Work out the finished part from the listing and answer in its coordinate system (mm). A direction names the side the tool comes from. Coordinates: 2 decimals unless noted, no trailing zeros. Loops run counter-clockwise (first coordinate to the right, second up) from the corner with the lowest first, then second, coordinate; pieces in that order, holes last. Notation, with made-up numbers: (18.25, 83) - (62.25, 83) arc R29 ccw to (62.25, 107) - close; hole circle Ø3 at (2, 30). An arc over 180 degrees is marked (long way). Write each question's results on one line, items separated by ' | '. Start each with the question number.
Item 1: Each of these flat-tipped pins is pushed along its axis until it touches: pin 1 Ø1 at (y, z) = (20, 1) entering from +X; pin 2 Ø3 at (x, z) = (101, 3.5) entering from -Y. Where does it stop, or does it pass through?
Item 2: Consider probe 1 along X at (y, z) = (67.5, 4.9); probe 2 along X at (y, z) = (36.5, 1.3); probe 3 along X at (y, z) = (90.29, 2.85). Determine where each line is inside the solid, lowest interval first. Write a range as [from, to].
Item 3: Section A-A, the plane x = 69 is taken. Write down the section's boundary in (y, z) (3 decimals), plus the area to 4 significant figures.
Item 4: A tool of negligible diameter and unlimited length cuts with its end or side. For faces 1 (the face through (145, 16.73, 3)), 2 (the face through (35, 90.73, 3)), 3 (the face through (-89, -35, 3)), from which of +Z, -Z, +X, -X, +Y, -Y can it reach the whole face along a straight path? Write none if from no direction.
Item 5: Section C-C, the plane z = 1.05 is taken. Count the separate pieces of the cut face and the enclosed holes in it, plus the area to 3 significant figures.
Item 6: For a pull along Y with two mould halves and no side action, classify faces 4 (the face through (-109, -35, 3)), 5 (the face through (-162, 83.853, 3)), 6 (the face through (-105, 90.73, 3)) as +Y half, -Y half, draft (parallel to the pull), parting line (faces both ways), or undercut.
Item 7: Section B-B, the plane y = 31 is taken. Write down the section's boundary in (x, z), plus the area to 3 significant figures.
from build123d import *

# Parameters (mm, degrees)
BOSS_EXTRU_1_DEPTH      = 6
ESQUISSE3_W             = 6
ESQUISSE3_H             = 10
ESQUISSE3_W_2           = 20
ESQUISSE3_H_2           = 6
ESQUISSE3_W_3           = 60
ESQUISSE3_H_3           = 110
ESQUISSE3_W_4           = 40
ESQUISSE3_H_4           = 20
ENL_V_MAT_EXTRU_2_DEPTH = 6
ESQUISSE4_R             = 1.5
ENL_V_MAT_EXTRU_3_DEPTH = 6
ESQUISSE5_W             = 456.045253014
ESQUISSE5_H             = 136.228984631
ENL_V_MAT_EXTRU_4_DEPTH = 6


with BuildPart() as part:
    # Esquisse1 → Boss.-Extru.1 (new body)
    with BuildSketch(Plane.XY):
        Polygon((-165, 96.73), (165, 96.73), (165, -18.27), (123, -109.022410436), (-123, -109.022410436), (-165, -18.27), align=None)
    extrude(amount=BOSS_EXTRU_1_DEPTH)

    # Esquisse3 → Enlèv. mat.-Extru.2 (cut)
    with BuildSketch(Plane(origin=(0, 0, 0), x_dir=(-1, 0, 0), z_dir=(0, 0, -1))):
        with Locations((162, -4.85)):
            Rectangle(ESQUISSE3_W, ESQUISSE3_H)
        with Locations((162, 78.852589564)):
            Rectangle(ESQUISSE3_W, ESQUISSE3_H)
        with Locations((-24, -35.02)):
            Rectangle(ESQUISSE3_W_2, ESQUISSE3_H_2)
        with Locations((99, -35.02)):
            Rectangle(ESQUISSE3_W_2, ESQUISSE3_H_2)
        with Locations((-162, 51.23)):
            Rectangle(ESQUISSE3_W, ESQUISSE3_H)
        with Locations((-80, 29.355)):
            Rectangle(ESQUISSE3_W_3, ESQUISSE3_H_3)
        with Locations((24, -35.02)):
            Rectangle(ESQUISSE3_W_2, ESQUISSE3_H_2)
        with Locations((-162, 78.852589564)):
            Rectangle(ESQUISSE3_W, ESQUISSE3_H)
        with Locations((-162, -4.85)):
            Rectangle(ESQUISSE3_W, ESQUISSE3_H)
        with Locations((105, 93.73)):
            Rectangle(ESQUISSE3_W_2, ESQUISSE3_H_2)
        with Locations((-35, 93.73)):
            Rectangle(ESQUISSE3_W_2, ESQUISSE3_H_2)
        with Locations((35, 93.73)):
            Rectangle(ESQUISSE3_W_2, ESQUISSE3_H_2)
        with Locations((-105, 93.73)):
            Rectangle(ESQUISSE3_W_2, ESQUISSE3_H_2)
        with Locations((162, 51.23)):
            Rectangle(ESQUISSE3_W, ESQUISSE3_H)
        with Locations((-99, -35.02)):
            Rectangle(ESQUISSE3_W_2, ESQUISSE3_H_2)
        with Locations((-145, 26.73)):
            Rectangle(ESQUISSE3_W_4, ESQUISSE3_H_4)
        with Locations((145, 26.73)):
            Rectangle(ESQUISSE3_W_4, ESQUISSE3_H_4)
    extrude(amount=-ENL_V_MAT_EXTRU_2_DEPTH, mode=Mode.SUBTRACT)

    # Esquisse4 → Enlèv. mat.-Extru.3 (cut)
    with BuildSketch(Plane(origin=(0, 0, 0), x_dir=(-1, 0, 0), z_dir=(0, 0, -1))):
        with Locations((162, 7.65)):
            Circle(ESQUISSE4_R)
        with Locations((114, -35.02)):
            Circle(ESQUISSE4_R)
        with Locations((162, 65.042589564)):
            Circle(ESQUISSE4_R)
        with Locations((84, -35.02)):
            Circle(ESQUISSE4_R)
        with Locations((39, -35.02)):
            Circle(ESQUISSE4_R)
        with Locations((162, 90.29)):
            Circle(ESQUISSE4_R)
        with Locations((9, -35.02)):
            Circle(ESQUISSE4_R)
        with Locations((-9, -35.02)):
            Circle(ESQUISSE4_R)
        with Locations((-39, -35.02)):
            Circle(ESQUISSE4_R)
        with Locations((-84, -35.02)):
            Circle(ESQUISSE4_R)
        with Locations((120, 93.73)):
            Circle(ESQUISSE4_R)
        with Locations((-114, -35.02)):
            Circle(ESQUISSE4_R)
        with Locations((90, 93.73)):
            Circle(ESQUISSE4_R)
        with Locations((50, 93.73)):
            Circle(ESQUISSE4_R)
        with Locations((20, 93.73)):
            Circle(ESQUISSE4_R)
        with Locations((-20, 93.73)):
            Circle(ESQUISSE4_R)
        with Locations((-50, 93.73)):
            Circle(ESQUISSE4_R)
        with Locations((-90, 93.73)):
            Circle(ESQUISSE4_R)
        with Locations((-120, 93.73)):
            Circle(ESQUISSE4_R)
        with Locations((-162, 90.29)):
            Circle(ESQUISSE4_R)
        with Locations((-162, 65.042589564)):
            Circle(ESQUISSE4_R)
        with Locations((-162, 7.65)):
            Circle(ESQUISSE4_R)
    extrude(amount=-ENL_V_MAT_EXTRU_3_DEPTH, mode=Mode.SUBTRACT)

    # Esquisse5 → Enlèv. mat.-Extru.4 (cut)
    with BuildSketch(Plane(origin=(0, 0, 0), x_dir=(-1, 0, 0), z_dir=(0, 0, -1))):
        with Locations((-18.307092018, -106.134492316)):
            Rectangle(ESQUISSE5_W, ESQUISSE5_H)
    extrude(amount=-ENL_V_MAT_EXTRU_4_DEPTH, mode=Mode.SUBTRACT)


solid = part.part
Answer key:
1) pin 1: stops at x = 125 | pin 2: stops at y = -32.02
2) probe 1: x = [-165, 50], [110, 165] | probe 2: x = [-125, 50], [110, 125] | probe 3: x = [-165, -163.5], [-160.5, 160.5], [163.5, 165]
3) outline: (-38.02, 0) - (-25.645, 0) - (-25.645, 6) - (-38.02, 6) - close; (84.355, 0) - (96.73, 0) - (96.73, 6) - (84.355, 6) - close | area: 148.5 mm^2
4) face 1: +Z, -Z, +X | face 2: +Z, -Z, +Y | face 3: +Z, -Z, -Y
5) separate pieces: 1 | enclosed holes: 23 | area: 34,600 mm^2
6) face 4: draft | face 5: undercut | face 6: +Y half
7) outline: (-125, 0) - (50, 0) - (50, 6) - (-125, 6) - close; (110, 0) - (125, 0) - (125, 6) - (110, 6) - close | area: 1,140 mm^2
